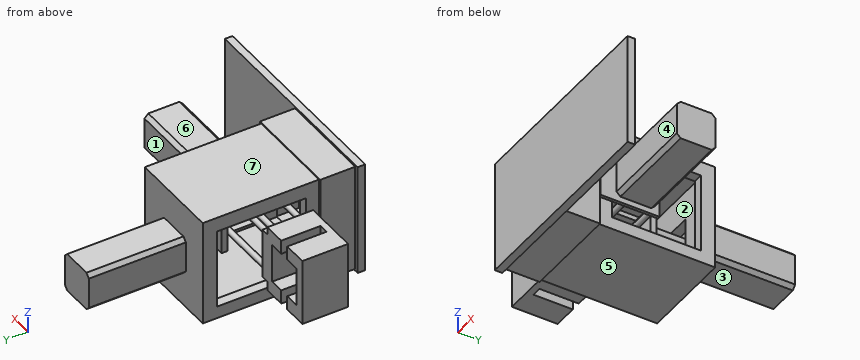
from build123d import *

# Parameters (mm, degrees)
SKETCH1_W            = 279.4
SKETCH1_H            = 147.32
BOSS_EXTRUDE1_DEPTH  = 10
SKETCH2_W            = 127
SKETCH2_H            = 142.24
BOSS_EXTRUDE2_DEPTH  = 45.72
SKETCH3_W            = 121.92
SKETCH3_H            = 139.7
BOSS_EXTRUDE3_DEPTH  = 152.4
SHELL1_START         = -130.81
SHELL1_DEPTH         = 114.3
SHELL1_START_2       = -132.08
SHELL1_2_OUTLINE_W   = 101.6
SHELL1_2_OUTLINE_H   = 30.32
SHELL1_2_DEPTH       = 116.84
SKETCH5_W            = 104.57255138
SKETCH5_H            = 116.526725643
CUT_EXTRUDE1_DEPTH   = 152.4
CUT_EXTRUDE2_REACH   = 380.261
SKETCH6_W            = 38.1
SKETCH6_H            = 38.1
SKETCH7_W            = 50.8
SKETCH7_H            = 50.8
BOSS_EXTRUDE4_DEPTH  = 127
SKETCH8_R            = 6.35
BOSS_EXTRUDE5_DEPTH  = 50.8
SKETCH9_W            = 38.1
SKETCH9_H            = 38.1
BOSS_EXTRUDE6_DEPTH  = 7.62
CHAMFER1_SIZE        = 5.08
SKETCH11_W           = 65.909153677
SKETCH11_H           = 77.291627037
BOSS_EXTRUDE8_DEPTH  = 3.81
SKETCH12_W           = 50.8
SKETCH12_H           = 50.8
BOSS_EXTRUDE9_DEPTH  = 127
CHAMFER2_SIZE        = 5.08
SKETCH13_R           = 3.81
BOSS_EXTRUDE10_DEPTH = 127
SKETCH14_W           = 65.909153677
SKETCH14_H           = 59.998529599
BOSS_EXTRUDE11_DEPTH = 10.16
SKETCH15_W           = 87.63
SKETCH15_H           = 59.998529599
BOSS_EXTRUDE12_DEPTH = 10.16
BOSS_EXTRUDE13_DEPTH = 19.05
SKETCH17_W           = 87.63
SKETCH17_H           = 8.552313921
BOSS_EXTRUDE14_DEPTH = 12.7
BOSS_EXTRUDE15_DEPTH = 19.05
SKETCH19_W           = 87.63
SKETCH19_H           = 59.998529599
BOSS_EXTRUDE16_DEPTH = 12.7


# Read off the part's stored shape, not the designer's step: Shell1
with BuildPart() as part:
    # Sketch1 → Boss-Extrude1 (new body)
    with BuildSketch(Plane(origin=(0, 0, 0), x_dir=(1, 0, 0), z_dir=(0, 1, 0))):
        with Locations((139.7, 73.66)):
            Rectangle(SKETCH1_W, SKETCH1_H)
    extrude(amount=BOSS_EXTRUDE1_DEPTH)

    # Sketch2 → Boss-Extrude2 (add)
    with BuildSketch(Plane(origin=(0, 10, 0), x_dir=(1, 0, 0), z_dir=(0, 1, 0))):
        with Locations((68.541128652, 73.66)):
            Rectangle(SKETCH2_W, SKETCH2_H)
    extrude(amount=BOSS_EXTRUDE2_DEPTH)

    # Sketch3 → Boss-Extrude3 (add)
    with BuildSketch(Plane(origin=(0, 55.72, 0), x_dir=(1, 0, 0), z_dir=(0, 1, 0))):
        with Locations((68.541128652, 73.66)):
            Rectangle(SKETCH3_W, SKETCH3_H)
    extrude(amount=BOSS_EXTRUDE3_DEPTH)

    # Shell1 outline → Shell1 (cut)
    with BuildSketch(Plane.XY.offset(SHELL1_START)):
        Polygon((17.741128652, 12.7), (119.341128652, 12.7), (119.341128652, 43.02), (116.801128652, 43.02), (116.801128652, 195.42), (20.281128652, 195.42), (20.281128652, 43.02), (17.741128652, 43.02), align=None)
    extrude(amount=SHELL1_DEPTH, mode=Mode.SUBTRACT)

    # Shell1 2 outline → Shell1 2 (cut)
    with BuildSketch(Plane.XY.offset(SHELL1_START_2)):
        with Locations((68.541128652, 27.86)):
            Rectangle(SHELL1_2_OUTLINE_W, SHELL1_2_OUTLINE_H)
    extrude(amount=SHELL1_2_DEPTH, mode=Mode.SUBTRACT)

    # Sketch5 → Cut-Extrude1 (cut)
    with BuildSketch(Plane(origin=(129.501128652, 0, 0), x_dir=(0, 0, -1), z_dir=(1, 0, 0))):
        with Locations((75.203066098, 131.276460259)):
            Rectangle(SKETCH5_W, SKETCH5_H)
    extrude(amount=-CUT_EXTRUDE1_DEPTH, mode=Mode.SUBTRACT)

    # Sketch6 → Cut-Extrude2 (cut, up to next)
    with BuildSketch(Plane(origin=(0, 208.12, 0), x_dir=(1, 0, 0), z_dir=(0, 1, 0)), mode=Mode.PRIVATE) as cut_extrude2_sk1:
        with Locations((68.541128652, 73.66)):
            Rectangle(SKETCH6_W, SKETCH6_H)
    cut_extrude2_tool1 = extrude(cut_extrude2_sk1.sketch, amount=-CUT_EXTRUDE2_REACH, mode=Mode.PRIVATE) & part.part
    add(cut_extrude2_tool1.solids().sort_by_distance((68.541129, 208.12, -73.66))[0], mode=Mode.SUBTRACT)

    # Sketch7 → Boss-Extrude4 (add)
    with BuildSketch(Plane(origin=(0, 208.12, 0), x_dir=(1, 0, 0), z_dir=(0, 1, 0))):
        with Locations((68.541128652, 73.66)):
            Rectangle(SKETCH7_W, SKETCH7_H)
    extrude(amount=BOSS_EXTRUDE4_DEPTH)

    # Sketch8 → Boss-Extrude5 (add)
    with BuildSketch(Plane.XZ.offset(-208.12)):
        with Locations(Location((68.541128652, -73.66, 0), (0, 0, 90))):
            Circle(SKETCH8_R)
    extrude(amount=BOSS_EXTRUDE5_DEPTH)

    # Sketch9 → Boss-Extrude6 (add)
    with BuildSketch(Plane.XZ.offset(-157.32)):
        with Locations((68.541128652, -73.66)):
            Rectangle(SKETCH9_W, SKETCH9_H)
    extrude(amount=BOSS_EXTRUDE6_DEPTH)

    # Chamfer1
    chamfer1_edges = [part.edges().sort_by_distance(p)[0] for p in [
        (43.141128652, 271.62, -99.06),
        (43.141128652, 271.62, -48.26),
        (93.941128652, 271.62, -48.26),
        (93.941128652, 271.62, -99.06),
    ]]
    chamfer(chamfer1_edges, length=CHAMFER1_SIZE)

    # Sketch11 → Boss-Extrude8 (add)
    with BuildSketch(Plane(origin=(129.501128652, 0, 0), x_dir=(0, 0, -1), z_dir=(1, 0, 0))):
        with Locations((72.491397984, 94.365813519)):
            Rectangle(SKETCH11_W, SKETCH11_H)
    extrude(amount=BOSS_EXTRUDE8_DEPTH)

    # Sketch12 → Boss-Extrude9 (add)
    with BuildSketch(Plane(origin=(133.311128652, 0, 0), x_dir=(0, 0, -1), z_dir=(1, 0, 0))):
        with Locations((72.356136011, 101.821276894)):
            Rectangle(SKETCH12_W, SKETCH12_H)
    extrude(amount=BOSS_EXTRUDE9_DEPTH)

    # Chamfer2
    chamfer2_edges = [part.edges().sort_by_distance(p)[0] for p in [
        (196.811128652, 127.221276894, -46.956136011),
        (196.811128652, 76.421276894, -46.956136011),
        (196.811128652, 76.421276894, -97.756136011),
        (196.811128652, 127.221276894, -97.756136011),
    ]]
    chamfer(chamfer2_edges, length=CHAMFER2_SIZE)

    # Sketch13 → Boss-Extrude10 (add)
    with BuildSketch(Plane.ZY.offset(-129.501128652)):
        with Locations(Location((-97.260941216, 125.126689221, 0), (0, 0, 180))):
            Circle(SKETCH13_R)
        with Locations(Location((-47.633379276, 125.126689221, 0), (0, 0, 180))):
            Circle(SKETCH13_R)
        with Locations(Location((-97.260941216, 80.811309035, 0), (0, 0, 180))):
            Circle(SKETCH13_R)
        with Locations(Location((-47.633379276, 80.811309035, 0), (0, 0, 180))):
            Circle(SKETCH13_R)
    extrude(amount=BOSS_EXTRUDE10_DEPTH)

    # Sketch14 → Boss-Extrude11 (add)
    with BuildSketch(Plane.ZY.offset(-2.501128652)):
        with Locations((-72.491397984, 103.012362238)):
            Rectangle(SKETCH14_W, SKETCH14_H)
    extrude(amount=BOSS_EXTRUDE11_DEPTH)

    # Sketch15 → Boss-Extrude12 (add)
    with BuildSketch(Plane.ZY.offset(7.658871348)):
        with Locations((-73.497023893, 103.012362238)):
            Rectangle(SKETCH15_W, SKETCH15_H)
    extrude(amount=BOSS_EXTRUDE12_DEPTH)

    # Sketch16 → Boss-Extrude13 (add)
    with BuildSketch(Plane.ZY.offset(17.818871348)):
        Polygon((-117.312023893, 133.011627037), (-98.897023893, 133.011627037), (-98.897023893, 81.565411359), (-48.097023893, 81.565411359), (-48.097023893, 133.011627037), (-29.682023893, 133.011627037), (-29.682023893, 73.013097438), (-117.312023893, 73.013097438), align=None)
    extrude(amount=BOSS_EXTRUDE13_DEPTH)

    # Sketch17 → Boss-Extrude14 (add)
    with BuildSketch(Plane.ZY.offset(36.868871348)):
        with Locations((-73.497023893, 77.289254399)):
            Rectangle(SKETCH17_W, SKETCH17_H)
    extrude(amount=BOSS_EXTRUDE14_DEPTH)

    # Sketch18 → Boss-Extrude15 (add)
    with BuildSketch(Plane.ZY.offset(49.568871348)):
        Polygon((-117.312023893, 73.013097438), (-117.312023893, 133.011627037), (-98.897023893, 133.011627037), (-98.897023893, 81.565411359), (-48.097023893, 81.565411359), (-48.097023893, 133.011627037), (-29.682023893, 133.011627037), (-29.682023893, 73.013097438), align=None)
    extrude(amount=BOSS_EXTRUDE15_DEPTH)

    # Sketch19 → Boss-Extrude16 (add)
    with BuildSketch(Plane.ZY.offset(68.618871348)):
        with Locations((-73.497023893, 103.012362238)):
            Rectangle(SKETCH19_W, SKETCH19_H)
    extrude(amount=BOSS_EXTRUDE16_DEPTH)


solid = part.part
Verification items for the finished model (mm, model axes). Face numbers are marked on the shaded views. A direction names the side the tool comes from. Coordinates: 2 decimals unless noted, no trailing zeros. Order: outer loops, then holes, each group sorted by start corner. A loop starts at its lowest first (then second) coordinate and runs counter-clockwise, first axis right, second up. Notation, with made-up numbers: M 55.25,56 L 91.25,56 A30 cw 91.25,93 Z; hole C -12.5,5.5 d5. An arc over 180 degrees is marked long. Write each question's results on one line, items separated by ' | '.
1) Access from +Z, -Z, +X, -X, +Y, -Y to the whole of each face (thin tool, end or side, straight path). Record for the marked faces 4, 5, 6 and 7.
Solved:
face 4: +Z, -Z, +X | face 5: -Z, +X, -X, +Y | face 6: +Z, +X, +Y | face 7: +Z, +X, -X, +Y
2) Section check A-A on x = 212.5. Record the cut outline in (y, z).
Solved:
outline: M 0,-147.32 L 10,-147.32 L 10,0 L 0,0 Z; M 76.42,-92.68 L 81.5,-97.76 L 122.14,-97.76 L 127.22,-92.68 L 127.22,-52.04 L 122.14,-46.96 L 81.5,-46.96 L 76.42,-52.04 Z
3) Gauge pin test, flat ends, axial feed: pin 1 Ø3 at (y, z) = (102.5, -34) entering from +X; pin 2 Ø2 at (x, z) = (210.5, -106.5) entering from -Y; pin 3 Ø8 at (x, y) = (-1, 111.5) entering from +Z; pin 4 Ø4 at (x, y) = (72, 154.5) entering from +Z. Record the tip position at first contact, or that the pin passes through.
Solved:
pin 1: stops at x = -7.66 | pin 2: stops at y = 0 | pin 3: stops at z = -39.54 | pin 4: stops at z = -3.81
4) Scan lines: line 1 along Y through (x, z) = (57, -90.5); line 2 along X through (y, z) = (77.5, -102.5); line 3 along Y through (x, z) = (97, -75.5). Record each from-to range of solid material in increasing order. Write a range as [from, to].
Solved:
line 1: y = [0, 12.7], [149.7, 157.32], [208.12, 335.12] | line 2: x = [-81.32, 2.5], [129.5, 133.31] | line 3: y = [0, 12.7], [195.42, 208.12]
5) Section check B-B on y = 229.5. Record the cut outline in (x, z).
Solved:
outline: M 43.14,-93.98 L 48.22,-99.06 L 88.86,-99.06 L 93.94,-93.98 L 93.94,-53.34 L 88.86,-48.26 L 48.22,-48.26 L 43.14,-53.34 Z
6) Release check for a two-part mould opening along Y. For the marked faces 1, 2 and 3 record: pulls with the +Y half, pulls with the -Y half, needs draft (parallel to the pull), parting line crosses it, or undercut.
Solved:
face 1: pulls with the +Y half | face 2: undercut | face 3: needs draft
7) Section check D-D on y = 97. Give the number of separate pieces and of enclosed holes in the cut face, plus the area to 3 significant figures.
Solved:
separate pieces: 5 | enclosed holes: 0 | area: 14,100 mm²
8) Section check C-C on x = 108.5. Record the cut outline in (y, z).
Solved:
outline: M 0,-147.32 L 10,-147.32 L 10,-144.78 L 55.72,-144.78 L 55.72,-143.51 L 208.12,-143.51 L 208.12,-3.81 L 55.72,-3.81 L 55.72,-2.54 L 10,-2.54 L 10,0 L 0,0 Z; C 80.81,-97.26 d7.62; C 80.81,-47.63 d7.62; C 125.13,-97.26 d7.62; C 125.13,-47.63 d7.62; hole M 12.7,-132.08 L 43.02,-132.08 L 43.02,-130.81 L 195.42,-130.81 L 195.42,-16.51 L 43.02,-16.51 L 43.02,-15.24 L 12.7,-15.24 Z
